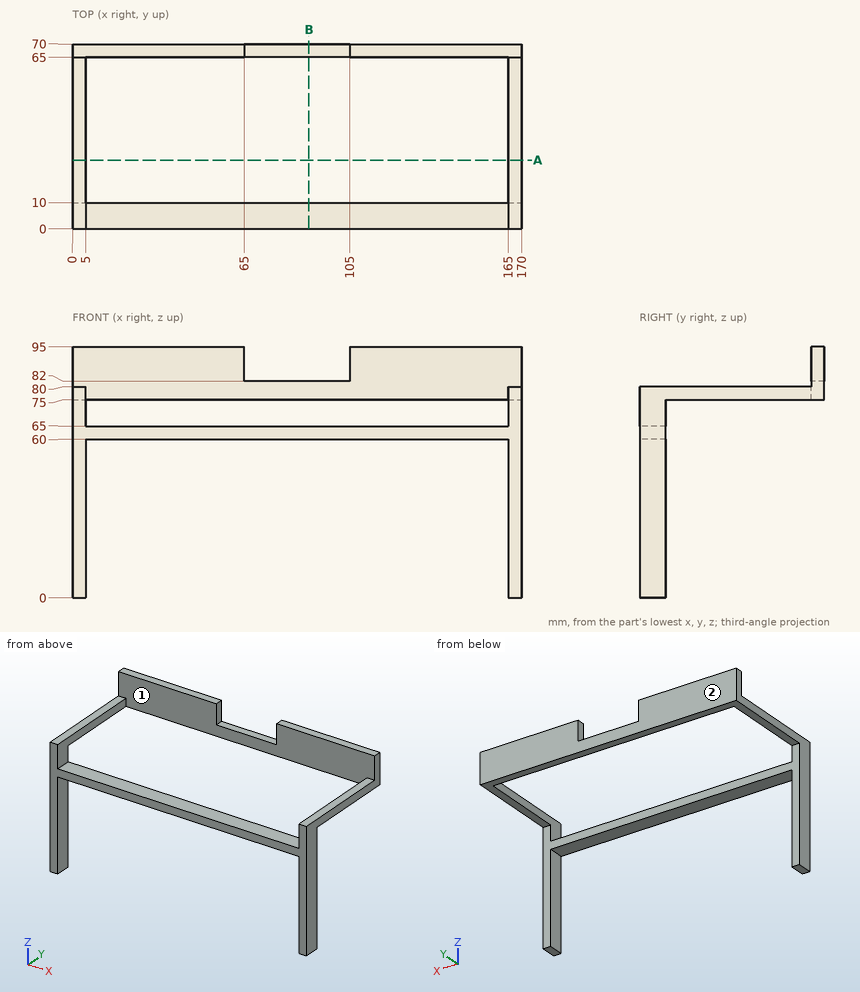
Drawing for the job (mm, zero at the part's lowest x, y, z). Give positions to 0.01 mm unless a question says otherwise; leave off trailing zeros. Loops run counter-clockwise (first coordinate to the right, second up) from the corner with the lowest first, then second, coordinate; pieces in that order, holes last.
(1) Band-saw the part on B-B (x = 89.5). Write the cut outline in (y, z), and give its area (3 significant figures).
Return value:
outline: (0, 60) - (10, 60) - (10, 65) - (0, 65) - close; (65, 75) - (70, 75) - (70, 82) - (65, 82) - close
area: 85.0 mm2
(2) Pull direction X, two halves, no side cores. Call the marked faces 1 and 2: pulls with the +X half, pulls with the -X half, needs draft (parallel to the pull), parting line crosses it, or undercut.
Return value:
face 1: undercut
face 2: needs draft
(3) Band-saw the part on A-A (y = 26). Write the cut outline in (x, z), and give its area (3 significant figures).
Return value:
outline: (0, 75) - (5, 75) - (5, 80) - (0, 80) - close; (165, 75) - (170, 75) - (170, 80) - (165, 80) - close
area: 50.0 mm2
(4) Drill centre lines: line 1 along X through (y, z) = (3, 70); line 2 along Z through (x, y) = (111, 5.5). Where is each one in solid material? Low to high.
Return value:
line 1: x = 0 to 5, 165 to 170
line 2: z = 60 to 65
(5) Pin check, flat tips, straight feed: pin 1 (4 mm diameter, centred on x = 91, y = 68, fed in from +Z); pin 2 (22 mm diameter, centred on x = 79.5, z = 82, fed in from -Y); pin 3 (2.5 mm diameter, centred on x = 168.5, y = 39, fed in from +Z); pin 4 (5 mm diameter, centred on y = 7.5, z = 41.5, fed in from -X). Stop position of each tip, or through.
Return value:
pin 1: stops at z = 82
pin 2: stops at y = 65
pin 3: stops at z = 80
pin 4: stops at x = 0
